from build123d import *

# Parameters (mm, degrees)
SKETCH1_R           = 31
SKETCH1_R_2         = 15
BOSS_EXTRUDE1_DEPTH = 20
SKETCH2_R           = 28.2
SKETCH2_R_2         = 18.25
CUT_EXTRUDE1_DEPTH  = 0.5
SKETCH3_R           = 28.2
SKETCH3_R_2         = 18.25
CUT_EXTRUDE2_DEPTH  = 0.5


with BuildPart() as part:
    # Sketch1 → Boss-Extrude1 (new body)
    with BuildSketch(Plane(origin=(0, 0, 0), x_dir=(1, 0, 0), z_dir=(0, 1, 0))):
        Circle(SKETCH1_R)
        Circle(SKETCH1_R_2, mode=Mode.SUBTRACT)
    extrude(amount=BOSS_EXTRUDE1_DEPTH)

    # Sketch2 → Cut-Extrude1 (cut)
    with BuildSketch(Plane(origin=(0, 20, 0), x_dir=(1, 0, 0), z_dir=(0, 1, 0))):
        Circle(SKETCH2_R)
        Circle(SKETCH2_R_2, mode=Mode.SUBTRACT)
    extrude(amount=-CUT_EXTRUDE1_DEPTH, mode=Mode.SUBTRACT)

    # Sketch3 → Cut-Extrude2 (cut)
    with BuildSketch(Plane.XZ):
        Circle(SKETCH3_R)
        Circle(SKETCH3_R_2, mode=Mode.SUBTRACT)
    extrude(amount=-CUT_EXTRUDE2_DEPTH, mode=Mode.SUBTRACT)


solid = part.part
Can you work these out from the model? Positions are in its coordinate system, mm. A direction names the side the tool comes from. Round coordinates to 2 decimals unless told otherwise and drop trailing zeros. Loops run counter-clockwise (first coordinate to the right, second up) from the corner with the lowest first, then second, coordinate; pieces in that order, holes last. Notation, with made-up numbers: (19, 45.25) - (26, 45.25) arc R16 cw to (26, 58.25) - close; hole circle Ø11 at (57.5, 47). An arc over 180 degrees is marked (long way). Write item = value, one per line. Start each with the question number.
(1) For faces 1 (the face through (-3, 20, 15)), 2 (the face through (-3.956, 0.246, -17.816)), 3 (the face through (-3.956, 19.754, 17.816)), which set-ups out of +Z, -Z, +X, -X, +Y, -Y let a thin tool reach every point of the face, with its end or its side?
(2) If we mould it in two halves opening along Z, with no side actions, what happens to faces 4 (the face through (-4.036, 9.86, -30.736)), 5 (the face through (13.01, 0.25, -25.02)), 6 (the face through (-3, 0, 15))? For each: released by +Z, released by -Z, zero draft, split by the parting line, or undercut.
(3) If we section it at D-D (x = -20): Please give me the cut outline in (y, z), and give its area (3 significant figures).
(4) If we section it at A-A (z = 0): Please give me the cut outline in (x, y).
(5) If we section it at C-C (y = 6.75): Please give me the cut outline in (x, z), and give its area (3 significant figures).
(6) For P1, Ø5, axis at x = -23.5, y = 15.5, coming from the +Z side; P2, Ø1.5, axis at y = 14.5, z = 14.5, coming from the +X side; P3, Ø17, axis at x = -2, z = -6, coming from the -Y side (3 decimals); P4, Ø2, axis at x = -10.5, y = 4.5, coming from the -Z side, each with a flat end and sliding along its axis, tell me the tip position at first contact or that it passes through.
(7) If I drill on probe 1 along Z at (x, y) = (0, 19.6); probe 2 along X at (y, z) = (12.5, 0), over which ranges is the centre line in solid material (lowest first)? Write a range as [from, to].
(8) If we section it at B-B (x = 0): Please give me the cut outline in (y, z).
Ans:
q1.face_1 = +Z, -Z, +X, -X, +Y
q1.face_2 = -Y
q1.face_3 = +Y
q2.face_4 = split by the parting line
q2.face_5 = undercut
q2.face_6 = zero draft
q3.outline = (0, -23.69) - (20, -23.69) - (20, -19.88) - (19.5, -19.88) - (19.5, 19.88) - (20, 19.88) - (20, 23.69) - (0, 23.69) - (0, 19.88) - (0.5, 19.88) - (0.5, -19.88) - (0, -19.88) - close
q3.area = 908 mm²
q4.outline = (-31, 0) - (-28.2, 0) - (-28.2, 0.5) - (-18.25, 0.5) - (-18.25, 0) - (-15, 0) - (-15, 20) - (-18.25, 20) - (-18.25, 19.5) - (-28.2, 19.5) - (-28.2, 20) - (-31, 20) - close; (15, 0) - (18.25, 0) - (18.25, 0.5) - (28.2, 0.5) - (28.2, 0) - (31, 0) - (31, 20) - (28.2, 20) - (28.2, 19.5) - (18.25, 19.5) - (18.25, 20) - (15, 20) - close
q5.outline = circle Ø62 at (0, 0); hole circle Ø30 at (0, 0)
q5.area = 2,310 mm²
q6.P1 = 22.8
q6.P2 = 27.78
q6.P3 = through
q6.P4 = -29.51
q7.probe_1 = [-31, -28.2], [-18.25, -15], [15, 18.25], [28.2, 31]
q7.probe_2 = [-31, -15], [15, 31]
q8.outline = (0, -31) - (20, -31) - (20, -28.2) - (19.5, -28.2) - (19.5, -18.25) - (20, -18.25) - (20, -15) - (0, -15) - (0, -18.25) - (0.5, -18.25) - (0.5, -28.2) - (0, -28.2) - close; (0, 15) - (20, 15) - (20, 18.25) - (19.5, 18.25) - (19.5, 28.2) - (20, 28.2) - (20, 31) - (0, 31) - (0, 28.2) - (0.5, 28.2) - (0.5, 18.25) - (0, 18.25) - close
